Geometry: final body of the model. Coordinates: model frame, mm. Round coordinates to 2 decimals unless told otherwise and drop trailing zeros. Loops run counter-clockwise (first coordinate to the right, second up) from the corner with the lowest first, then second, coordinate; pieces in that order, holes last. Notation, with made-up numbers: (-34, -25) - (-19, -25) arc R29 cw to (-19, 7) - close; hole circle Ø8 at (-24.5, 68). An arc over 180 degrees is marked (long way). Use CSV: the item, a comma, the result in double quotes.
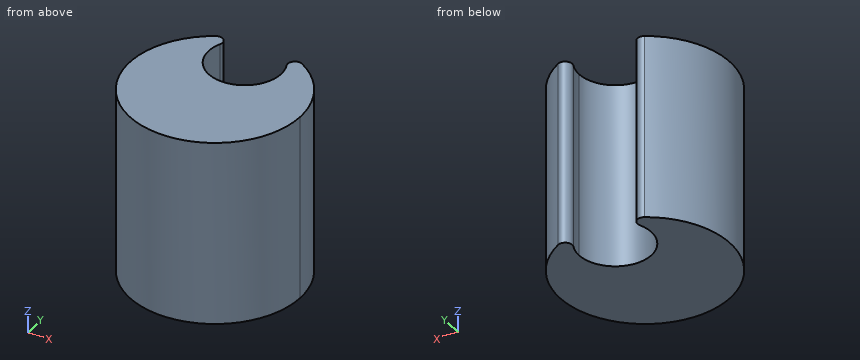
from build123d import *

# Parameters (mm, degrees)
AUFSATZ_LINEAR_AUSTRAGEN2_DEPTH = 13
VERRUNDUNG1_R                   = 0.5


with BuildPart() as part:
    # Skizze1 → Aufsatz-Linear austragen2 (new body)
    with BuildSketch(Plane.XY):
        with BuildLine():
            ThreePointArc((-0.771783993, 5.950155415), (-3.960384832, -4.507255482), (6, 0))
            ThreePointArc((6, 0), (4.507255482, 3.960384832), (0.771783993, 5.950155415))
            ThreePointArc((0.771783993, 5.950155415), (2.057978278, 5.025485179), (2.55, 3.519754323))
            ThreePointArc((2.55, 3.519754323), (-1.505730855, 1.461776046), (-0.771783993, 5.950155415))
        make_face()
    extrude(amount=AUFSATZ_LINEAR_AUSTRAGEN2_DEPTH)

    # Verrundung1
    verrundung1_edges = [part.edges().sort_by_distance(p)[0] for p in [
        (-0.771783993, 5.950155415, 6.5),
        (0.771783993, 5.950155415, 6.5),
    ]]
    fillet(verrundung1_edges, radius=VERRUNDUNG1_R)


solid = part.part
Item 1: Section A-A on x = 0. Return the cut outline in (y, z).
Final values:
outline,"(-6, 0) - (0.97, 0) - (0.97, 13) - (-6, 13) - close"
Item 2: Section B-B on y = -3.25. Return the cut outline in (x, z), plus the area to 3 significant figures.
Final values:
outline,"(-5.04, 0) - (5.04, 0) - (5.04, 13) - (-5.04, 13) - close"
area,"131 mm²"
Item 3: Pin query (flat end, axial travel): P1, Ø1.5, axis at y = 4, z = 11.5, coming from the -X side; P2, Ø1, axis at x = -0.5, y = 2.5, coming from the -Z side; P3, Ø4, axis at y = 2.5, z = 11.5, coming from the -X side. Return the tip coordinate at first contact, or that it passes through.
Final values:
P1,"stops at x = -5.04"
P2,"passes through"
P3,"stops at x = -5.98"
Item 4: Material intervals for line 1 (Y direction, x = 0, z = 9.5); line 2 (X direction, y = 2.75, z = 7.75); line 3 (X direction, y = 4, z = 4.5), sorted ascending.
Final values:
line 1,"y = -6 to 0.97"
line 2,"x = -5.33 to -2.43, 2.43 to 5.33"
line 3,"x = -4.47 to -2.5, 2.5 to 4.47"
